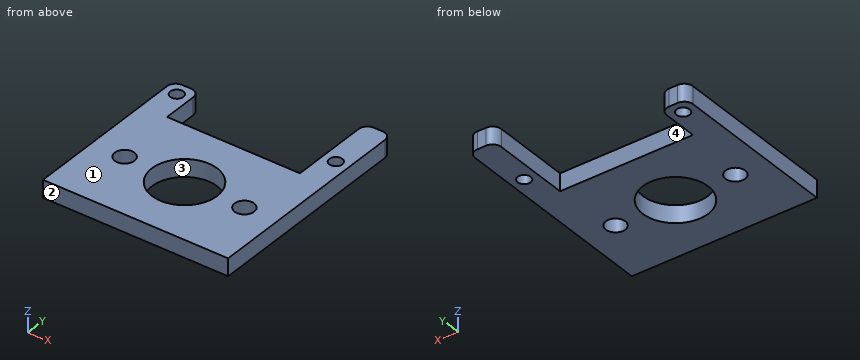
```python
from build123d import *

# Parameters (mm, degrees)
SKETCH_1_R      = 1.5
SKETCH_1_R_2    = 2.25
SKETCH_1_R_3    = 7.5
EXTRUDE_1_DEPTH = 4
FILLET_1_R      = 2


with BuildPart() as part:
    # 草图1 → 凸台-拉伸1 (new body)
    with BuildSketch(Plane.XY):
        Polygon((-18.007870082, 20.608843809), (-18.007870082, -13.606505187), (-18.007870082, -19.391156191), (24.492129918, -19.391156191), (24.492129918, 30.608843809), (18.492129918, 30.608843809), (18.492129918, 10.608843809), (-12.007870082, 10.608843809), (-12.007870082, 20.608843809), align=None)
        with Locations((-15.007870082, 17.608843809)):
            Circle(SKETCH_1_R, mode=Mode.SUBTRACT)
        with Locations((21.492129918, 17.608843809)):
            Circle(SKETCH_1_R, mode=Mode.SUBTRACT)
        with Locations((-10.507870082, -4.391156191)):
            Circle(SKETCH_1_R_2, mode=Mode.SUBTRACT)
        with Locations((16.992129918, -4.391156191)):
            Circle(SKETCH_1_R_2, mode=Mode.SUBTRACT)
        with Locations((3.242129918, -4.391156191)):
            Circle(SKETCH_1_R_3, mode=Mode.SUBTRACT)
    extrude(amount=EXTRUDE_1_DEPTH)

    # 圆角1
    fillet_1_edges = [part.edges().sort_by_distance(p)[0] for p in [
        (-12.007870082, 20.608843809, 2),
        (18.492129918, 30.608843809, 2),
        (24.492129918, 30.608843809, 2),
        (-18.007870082, 20.608843809, 2),
    ]]
    fillet(fillet_1_edges, radius=FILLET_1_R)


solid = part.part
```
Verification items for the finished model (mm, model axes). Face numbers are marked on the shaded views. Round coordinates to 2 decimals unless told otherwise and drop trailing zeros. Write each loop counter-clockwise with the first axis right and the second up, starting at its lowest first coordinate (ties: lowest second). Pieces come first, ordered by that corner, then holes. Notation, with made-up numbers: (28.25, 87.5) -> (67.25, 87.5) arc R24 cw to (67.25, 104.5) -> close; hole circle Ø7 at (-40, 60). An arc over 180 degrees is marked (long way). Write each question's results on one line, items separated by ' | '.
Q1. Sectioned sample at D-D, the plane y = -6. Record the boundary of the cut face in (x, z).
Derived:
outline: (-18.01, 0) -> (-12.08, 0) -> (-12.08, 4) -> (-18.01, 4) -> close; (-8.93, 0) -> (-4.08, 0) -> (-4.08, 4) -> (-8.93, 4) -> close; (10.57, 0) -> (15.42, 0) -> (15.42, 4) -> (10.57, 4) -> close; (18.57, 0) -> (24.49, 0) -> (24.49, 4) -> (18.57, 4) -> close
Q2. Sectioned sample at A-A, the plane y = 11.5. Record the boundary of the cut face in (x, z).
Derived:
outline: (-18.01, 0) -> (-12.01, 0) -> (-12.01, 4) -> (-18.01, 4) -> close; (18.49, 0) -> (24.49, 0) -> (24.49, 4) -> (18.49, 4) -> close
Q3. Go/stop test with flat-tipped pins: pin 1 Ø1.2 at (x, z) = (3, 2) entering from +Y; pin 2 Ø1.6 at (x, z) = (-15, 1.5) entering from +Y. Record where each tip stops, or that it passes through.
Derived:
pin 1: stops at y = 10.61 | pin 2: stops at y = 20.61
Q4. Draft check along Y on the marked faces 1, 2, 3 and 4. Enter one of: released by +Y, released by -Y, zero draft, split by the parting line, or undercut.
Derived:
face 1: zero draft | face 2: released by -Y | face 3: undercut | face 4: released by +Y
Q5. Thickness scan on probe 1 along X at (y, z) = (17.5, 3.65); probe 2 along X at (y, z) = (13.5, 1.5); probe 3 along X at (y, z) = (-3.5, 0.45). Record the ranges inside material, lowest first.
Derived:
probe 1: x = -18.01 to -16.5, -13.51 to -12.01, 18.49 to 20, 22.99 to 24.49 | probe 2: x = -18.01 to -12.01, 18.49 to 24.49 | probe 3: x = -18.01 to -12.57, -8.44 to -4.2, 10.69 to 14.93, 19.06 to 24.49
Q6. Sectioned sample at B-B, the plane x = -1. Record the boundary of the cut face in (y, z), and give its area (3 significant figures).
Derived:
outline: (-19.39, 0) -> (-10.58, 0) -> (-10.58, 4) -> (-19.39, 4) -> close; (1.79, 0) -> (10.61, 0) -> (10.61, 4) -> (1.79, 4) -> close | area: 70.5 mm²
Q7. Sectioned sample at C-C, the plane z = 1.7. Record the boundary of the cut face in (x, y).
Derived:
outline: (-18.01, -19.39) -> (24.49, -19.39) -> (24.49, 28.61) arc R2 ccw to (22.49, 30.61) -> (20.49, 30.61) arc R2 ccw to (18.49, 28.61) -> (18.49, 10.61) -> (-12.01, 10.61) -> (-12.01, 18.61) arc R2 ccw to (-14.01, 20.61) -> (-16.01, 20.61) arc R2 ccw to (-18.01, 18.61) -> close; hole circle Ø3 at (-15.01, 17.61); hole circle Ø4.5 at (-10.51, -4.39); hole circle Ø15 at (3.24, -4.39); hole circle Ø4.5 at (16.99, -4.39); hole circle Ø3 at (21.49, 17.61)
